from build123d import *

# Parameters (mm, degrees)
SKETCH_1_R      = 1.65
EXTRUDE_1_DEPTH = 5


with BuildPart() as part:
    # 草图1 → 凸台-拉伸1 (new body)
    with BuildSketch(Plane(origin=(0, 0, 0), x_dir=(1, 0, 0), z_dir=(0, 1, 0))):
        with BuildLine():
            Line((-75, 0), (0, -75))
            ThreePointArc((0, -75), (37.5, -90.533008589), (75, -75))
            ThreePointArc((75, -75), (86.496111183, -57.794853755), (90.533008589, -37.5))
            Line((90.533008589, -37.5), (90.533008589, 30.533008589))
            ThreePointArc((90.533008589, 30.533008589), (72.95941546, 72.95941546), (30.533008589, 90.533008589))
            Line((30.533008589, 90.533008589), (-37.5, 90.533008589))
            ThreePointArc((-37.5, 90.533008589), (-57.794853755, 86.496111183), (-75, 75))
            ThreePointArc((-75, 75), (-90.533008589, 37.5), (-75, 0))
        make_face()
        with Locations(Location((37.5, 65.5, 0), (0, 0, 270))):
            Circle(SKETCH_1_R, mode=Mode.SUBTRACT)
        with Locations(Location((61.748711306, 51.5, 0), (0, 0, 270))):
            Circle(SKETCH_1_R, mode=Mode.SUBTRACT)
        with Locations(Location((61.748711306, 23.5, 0), (0, 0, 270))):
            Circle(SKETCH_1_R, mode=Mode.SUBTRACT)
        with Locations(Location((37.5, 9.5, 0), (0, 0, 270))):
            Circle(SKETCH_1_R, mode=Mode.SUBTRACT)
        with Locations(Location((13.251288694, 23.5, 0), (0, 0, 270))):
            Circle(SKETCH_1_R, mode=Mode.SUBTRACT)
        with Locations(Location((13.251288694, 51.5, 0), (0, 0, 270))):
            Circle(SKETCH_1_R, mode=Mode.SUBTRACT)
        with Locations(Location((7.5, 67.5, 0), (0, 0, 270))):
            Circle(SKETCH_1_R, mode=Mode.SUBTRACT)
        with Locations(Location((67.5, 67.5, 0), (0, 0, 90))):
            Circle(SKETCH_1_R, mode=Mode.SUBTRACT)
        with Locations(Location((67.5, 7.5, 0), (0, 0, 270))):
            Circle(SKETCH_1_R, mode=Mode.SUBTRACT)
        with Locations(Location((7.5, 7.5, 0), (0, 0, 90))):
            Circle(SKETCH_1_R, mode=Mode.SUBTRACT)
        with Locations(Location((37.5, 37.5, 0), (0, 0, 270))):
            Circle(SKETCH_1_R, mode=Mode.SUBTRACT)
        with Locations(Location((-67.5, 67.5, 0), (0, 0, 270))):
            Circle(SKETCH_1_R, mode=Mode.SUBTRACT)
        with Locations(Location((-7.5, 67.5, 0), (0, 0, 270))):
            Circle(SKETCH_1_R, mode=Mode.SUBTRACT)
        with Locations(Location((-67.5, 7.5, 0), (0, 0, 270))):
            Circle(SKETCH_1_R, mode=Mode.SUBTRACT)
        with Locations(Location((-7.5, 7.5, 0), (0, 0, 270))):
            Circle(SKETCH_1_R, mode=Mode.SUBTRACT)
        with Locations(Location((7.5, -67.5, 0), (0, 0, 90))):
            Circle(SKETCH_1_R, mode=Mode.SUBTRACT)
        with Locations(Location((7.5, -7.5, 0), (0, 0, 90))):
            Circle(SKETCH_1_R, mode=Mode.SUBTRACT)
        with Locations(Location((67.5, -7.5, 0), (0, 0, 90))):
            Circle(SKETCH_1_R, mode=Mode.SUBTRACT)
        with Locations(Location((67.5, -67.5, 0), (0, 0, 90))):
            Circle(SKETCH_1_R, mode=Mode.SUBTRACT)
        with Locations(Location((-30, -30, 0), (0, 0, 270))):
            Circle(SKETCH_1_R, mode=Mode.SUBTRACT)
    extrude(amount=EXTRUDE_1_DEPTH)


solid = part.part
Check sheet for the modelled part. Datum: model origin and axes. Units: mm. Give positions to 0.01 mm unless a question says otherwise; leave off trailing zeros. Loops run counter-clockwise (first coordinate to the right, second up) from the corner with the lowest first, then second, coordinate; pieces in that order, holes last. Notation, with made-up numbers: M -29.75,77.5 L 6.25,77.5 A16 ccw 6.25,106.5 Z; hole C -10,86 d9. An arc over 180 degrees is marked long. Use a Markdown table: item, result. Add a question column.
Q1. Sectioned sample at A-A, the plane y = 4.1. Give the number of separate pieces and of enclosed holes in the cut face, then the cut area to 3 significant figures.
Q2. Scan lines: line 1 along X through (y, z) = (2.85, 6); line 2 along X through (y, z) = (2.8, -7.5); line 3 along Z through (x, y) = (12.5, 0.6). Record each from-to range of solid material in increasing order. Write a range as [from, to].
Q3. Mould release check, pull along X, two halves, no side actions. Record for faces 1 (the flat face through (90.533, 2, 4)), 2 (the flat face through (19, 5, -21)), 3 (the flat face through (-38, 2, 37)): pulls with the +X half, pulls with the -X half, needs draft (parallel to the pull), parting line crosses it, or undercut.
Q4. Go/stop test with a flat-tipped pin: pin 1 (2 mm diameter, centred on x = 61.75, z = -51.5, fed in from -Y). Record where the tip stops, or that it passes through.
Q5. Sectioned sample at B-B, the plane z = 14. Record the cut outline in (x, y), then the cut area to 3 significant figures.
Q6. Sectioned sample at C-C, the plane x = -41.5. Record the cut outline in (y, z), then the cut area to 3 significant figures.
Verdict:
| question | item | result |
|---|---|---|
| 1 | separate pieces | 1 |
| 1 | enclosed holes | 20 |
| 1 | area | 24,900 mm^2 |
| 2 | line 1 | [-69, 6.81], [8.19, 66.81], [68.19, 90.53] |
| 2 | line 2 | [-81.23, -69.15], [-65.85, -9.15], [-5.85, 5.85], [9.15, 65.85], [69.15, 90.53] |
| 2 | line 3 | [-90.53, -52.97], [-50.03, -24.97], [-22.03, 84.27] |
| 3 | face 1 | pulls with the +X half |
| 3 | face 2 | needs draft |
| 3 | face 3 | pulls with the -X half |
| 4 | pin 1 | through |
| 5 | outline | M -61,0 L 90.53,0 L 90.53,5 L -61,5 Z |
| 5 | area | 758 mm^2 |
| 6 | outline | M 0,-90.38 L 5,-90.38 L 5,33.5 L 0,33.5 Z |
| 6 | area | 619 mm^2 |
